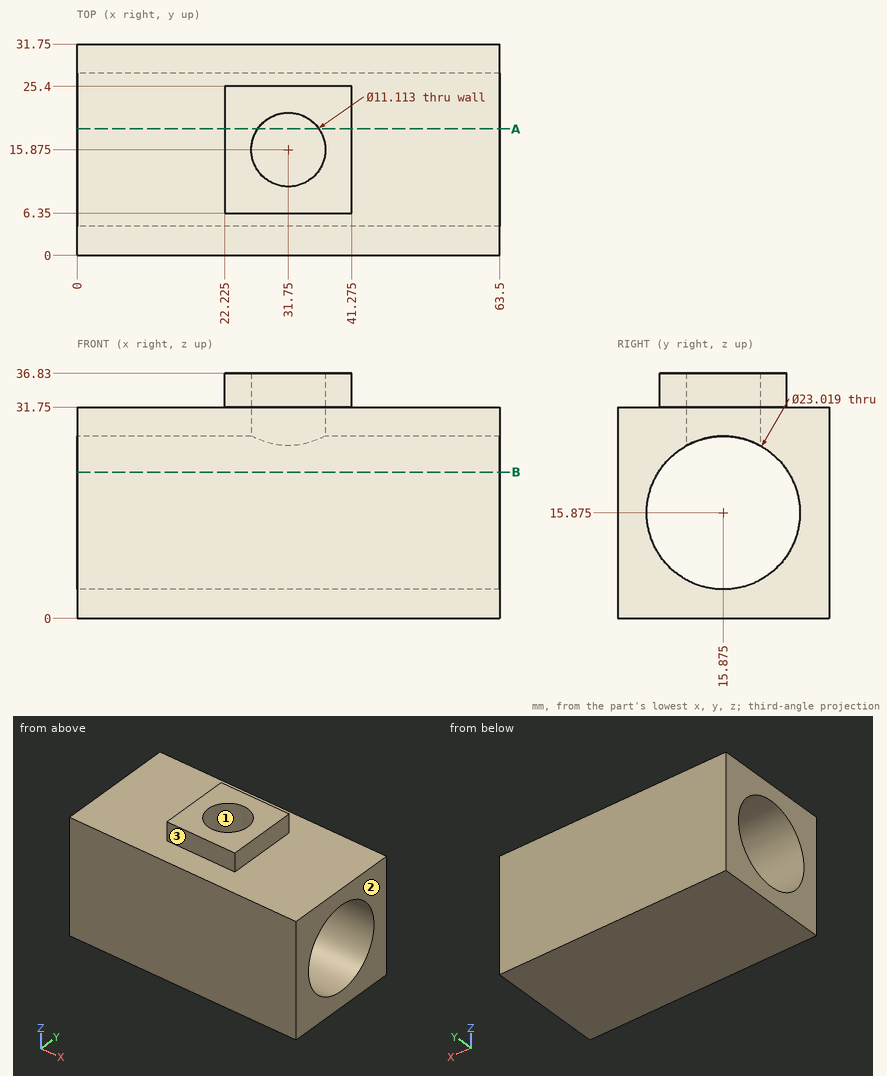
Drawing for the job (mm, zero at the part's lowest x, y, z). Give positions to 0.01 mm unless a question says otherwise; leave off trailing zeros. Loops run counter-clockwise (first coordinate to the right, second up) from the corner with the lowest first, then second, coordinate; pieces in that order, holes last. Notation, with made-up numbers: (34.5, 74) - (92.5, 74) arc R24 ccw to (92.5, 84) - close; hole circle Ø4 at (-18.5, -29). An arc over 180 degrees is marked (long way). Write item = value, one per line. Start each with the question number.
1) Pull direction Y, two halves, no side cores. Call the marked faces 1, 2 and 3: +Y half, -Y half, draft (parallel to the pull), parting line (faces both ways), or undercut.
2) Band-saw the part on B-B on z = 22. Give the cut face in (x, y).
3) Probe probe 1 along Y at (x, z) = (31.75, 29.75); probe 2 along Z at (x, y) = (31.5, 28); probe 3 along Y at (x, z) = (22, 11). List the from-to ranges inside material, lowest first. Write a range as from..to.
4) Band-saw the part on A-A on y = 19. Count the separate pieces of the cut face and the enclosed holes in it.
5) Drop flat-ended pins along their axis: pin 1 Ø2.5 at (y, z) = (18.5, 33.5) entering from +X (1 decimal); pin 2 Ø2.5 at (x, z) = (34, 33.5) entering from +Y. Give the stop position or say it passes through.
Final values:
q1.face_1 = undercut
q1.face_2 = draft
q1.face_3 = -Y half
q2.outline = (0, 0) - (63.5, 0) - (63.5, 6.13) - (0, 6.13) - close; (0, 25.62) - (63.5, 25.62) - (63.5, 31.75) - (0, 31.75) - close
q3.probe_1 = 0..10.32, 21.43..31.75
q3.probe_2 = 0..31.75
q3.probe_3 = 0..5.45, 26.3..31.75
q4.separate_pieces = 3
q4.enclosed_holes = 0
q5.pin_1 = 41.3
q5.pin_2 = 25.4
